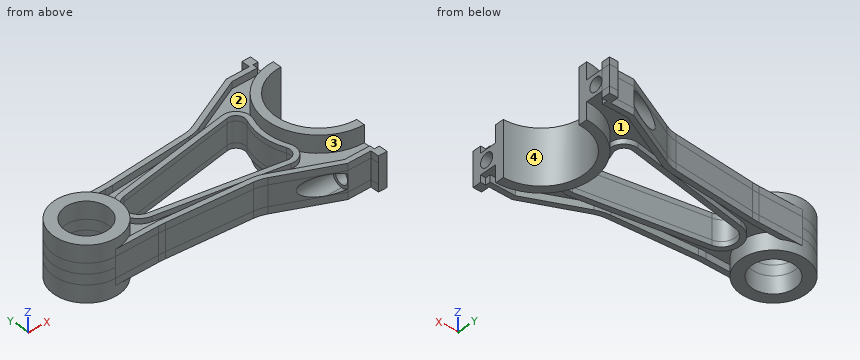
from build123d import *

# Parameters (mm, degrees)
SKETCH1_R           = 19
SKETCH1_R_2         = 12.5
BOSS_EXTRUDE1_DEPTH = 6
SKETCH1_4_R         = 19
SKETCH1_4_R_2       = 12.5
BOSS_EXTRUDE2_DEPTH = 16
BOSS_EXTRUDE3_DEPTH = 10
SKETCH3_R           = 4
CUT_EXTRUDE2_DEPTH  = 18.5
SKETCH4_R           = 5.795
CUT_EXTRUDE4_DEPTH  = 144.94417008
BOSS_EXTRUDE4_DEPTH = 9


with BuildPart() as part:
    # Sketch1 → Boss-Extrude1 (new, symmetric)
    # profile 1 of 3: a face of its own
    with BuildSketch(Plane.XY):
        with Locations((-135.29, 0)):
            Circle(SKETCH1_R)
        with Locations((-135.29, 0)):
            Circle(SKETCH1_R_2, mode=Mode.SUBTRACT)
    # profile 2 of 3: a face of its own
    with BuildSketch(Plane.XY):
        with BuildLine():
            Line((-110.00450535, 19), (-135.29, 19))
            ThreePointArc((-135.29, 19), (-121.854971157, 13.435028843), (-116.29, 0))
            ThreePointArc((-116.29, 0), (-121.854971157, -13.435028843), (-135.29, -19))
            Line((-135.29, -19), (-110.00450535, -19))
            ThreePointArc((-110.00450535, -19), (-108.041514562, -19.038548188), (-106.081550564, -19.154133313))
            Line((-106.081550564, -19.154133313), (-58.361460534, -22.909785849))
            ThreePointArc((-58.361460534, -22.909785849), (-54.838603484, -23.507213745), (-51.478277214, -24.721976782))
            Line((-51.478277214, -24.721976782), (-18.5, -40.1))
            Line((-18.5, -40.1), (-5, -40.1))
            Line((-5, -40.1), (-5, -45))
            Line((-5, -45), (0, -45))
            Line((0, -45), (0, -30))
            ThreePointArc((0, -30), (-30, 0), (0, 30))
            Line((0, 30), (0, 45))
            Line((0, 45), (-5, 45))
            Line((-5, 45), (-5, 40.1))
            Line((-5, 40.1), (-18.5, 40.1))
            Line((-18.5, 40.1), (-51.478277214, 24.721976782))
            ThreePointArc((-51.478277214, 24.721976782), (-54.838603484, 23.507213745), (-58.361460534, 22.909785849))
            Line((-58.361460534, 22.909785849), (-106.081550564, 19.154133313))
            ThreePointArc((-106.081550564, 19.154133313), (-108.041514562, 19.038548188), (-110.00450535, 19))
        make_face()
        with BuildLine():
            ThreePointArc((-106.341033016, -7.886801028), (-113, 0), (-106.341033016, 7.886801028))
            Line((-106.341033016, 7.886801028), (-35.770781366, 19.886220952))
            ThreePointArc((-35.770781366, 19.886220952), (-31.0052687, 18.051447358), (-30.336236293, 12.988947901))
            ThreePointArc((-30.336236293, 12.988947901), (-33, 0), (-30.336236293, -12.988947901))
            ThreePointArc((-30.336236293, -12.988947901), (-31.0052687, -18.051447358), (-35.770781366, -19.886220952))
            Line((-35.770781366, -19.886220952), (-106.341033016, -7.886801028))
        make_face(mode=Mode.SUBTRACT)
    # profile 3 of 3: a face of its own
    with BuildSketch(Plane.XY):
        with BuildLine():
            Line((0, 25), (0, 30))
            ThreePointArc((0, 30), (-30, 0), (0, -30))
            Line((0, -30), (0, -25))
            ThreePointArc((0, -25), (-25, 0), (0, 25))
        make_face()
    extrude(amount=BOSS_EXTRUDE1_DEPTH, both=True)

    # Sketch1_4 → Boss-Extrude2 (add, symmetric)
    # profile 1 of 2: a face of its own
    with BuildSketch(Plane.XY):
        with Locations((-135.29, 0)):
            Circle(SKETCH1_4_R)
        with Locations((-135.29, 0)):
            Circle(SKETCH1_4_R_2, mode=Mode.SUBTRACT)
    # profile 2 of 2: a face of its own
    with BuildSketch(Plane.XY):
        with BuildLine():
            Line((0, 25), (0, 30))
            ThreePointArc((0, 30), (-30, 0), (0, -30))
            Line((0, -30), (0, -25))
            ThreePointArc((0, -25), (-25, 0), (0, 25))
        make_face()
    extrude(amount=BOSS_EXTRUDE2_DEPTH, both=True)

    # Sketch2 → Boss-Extrude3 (add, symmetric)
    with BuildSketch(Plane.XY):
        with BuildLine():
            Line((-5, 45), (-5, 40.1))
            Line((-5, 40.1), (-18.5, 40.1))
            Line((-18.5, 40.1), (-51.478277214, 24.721976782))
            ThreePointArc((-51.478277214, 24.721976782), (-54.838603484, 23.507213745), (-58.361460534, 22.909785849))
            Line((-58.361460534, 22.909785849), (-106.081550564, 19.154133313))
            ThreePointArc((-106.081550564, 19.154133313), (-108.041514562, 19.038548188), (-110.00450535, 19))
            Line((-110.00450535, 19), (-135.29, 19))
            ThreePointArc((-135.29, 19), (-129.951460874, 18.234582529), (-125.043049234, 16))
            Line((-125.043049234, 16), (-110.00450535, 16))
            ThreePointArc((-110.00450535, 16), (-107.923735115, 16.040861079), (-105.846173277, 16.163381312))
            Line((-105.846173277, 16.163381312), (-58.126083247, 19.919033847))
            ThreePointArc((-58.126083247, 19.919033847), (-54.07479764, 20.606075928), (-50.210422429, 22.003053421))
            Line((-50.210422429, 22.003053421), (-17.834916012, 37.1))
            Line((-17.834916012, 37.1), (-3, 37.1))
            Line((-3, 37.1), (-3, 40))
            Line((-3, 40), (0, 40))
            Line((0, 40), (0, 45))
            Line((0, 45), (-5, 45))
        make_face()
        with BuildLine():
            Line((0, -40), (-3, -40))
            Line((-3, -40), (-3, -37.1))
            Line((-3, -37.1), (-17.834916012, -37.1))
            Line((-17.834916012, -37.1), (-50.210422429, -22.003053421))
            ThreePointArc((-50.210422429, -22.003053421), (-54.07479764, -20.606075928), (-58.126083247, -19.919033847))
            Line((-58.126083247, -19.919033847), (-105.846173277, -16.163381312))
            ThreePointArc((-105.846173277, -16.163381312), (-107.923735115, -16.040861079), (-110.00450535, -16))
            Line((-110.00450535, -16), (-125.043049234, -16))
            ThreePointArc((-125.043049234, -16), (-129.951460874, -18.234582529), (-135.29, -19))
            Line((-135.29, -19), (-110.00450535, -19))
            ThreePointArc((-110.00450535, -19), (-108.041514562, -19.038548188), (-106.081550564, -19.154133313))
            Line((-106.081550564, -19.154133313), (-58.361460534, -22.909785849))
            ThreePointArc((-58.361460534, -22.909785849), (-54.838603484, -23.507213745), (-51.478277214, -24.721976782))
            Line((-51.478277214, -24.721976782), (-18.5, -40.1))
            Line((-18.5, -40.1), (-5, -40.1))
            Line((-5, -40.1), (-5, -45))
            Line((-5, -45), (0, -45))
            Line((0, -45), (0, -40))
        make_face()
    extrude(amount=BOSS_EXTRUDE3_DEPTH, both=True)

    # Sketch3 → Cut-Extrude2 (cut)
    with BuildSketch(Plane(origin=(0, 0, 0), x_dir=(0, 0, -1), z_dir=(1, 0, 0))):
        with Locations(Location((0, -36, 0), (0, 0, 90))):
            Circle(SKETCH3_R)
    cut_extrude2 = extrude(amount=-CUT_EXTRUDE2_DEPTH, mode=Mode.SUBTRACT)

    # Sketch4 → Cut-Extrude4 (cut, through all)
    with BuildSketch(Plane(origin=(-18.5, 0, 0), x_dir=(0, 0, -1), z_dir=(1, 0, 0))):
        with Locations((0, -36)):
            Circle(SKETCH4_R)
    cut_extrude4 = extrude(amount=-CUT_EXTRUDE4_DEPTH, mode=Mode.SUBTRACT)

    # Mirror1: Cut-Extrude2, Cut-Extrude4 across plane
    add(cut_extrude2.mirror(Plane.ZX), mode=Mode.SUBTRACT)
    add(cut_extrude4.mirror(Plane.ZX), mode=Mode.SUBTRACT)

    # Sketch5 → Boss-Extrude4 (add, symmetric)
    with BuildSketch(Plane.XY):
        with BuildLine():
            Line((-106.843920397, 10.844351413), (-36.273668747, 22.843771338))
            ThreePointArc((-36.273668747, 22.843771338), (-28.648848481, 19.908133587), (-27.57839663, 11.808134455))
            ThreePointArc((-27.57839663, 11.808134455), (-30, 0), (-27.57839663, -11.808134455))
            ThreePointArc((-27.57839663, -11.808134455), (-28.648848481, -19.908133587), (-36.273668747, -22.843771338))
            Line((-36.273668747, -22.843771338), (-106.843920397, -10.844351413))
            ThreePointArc((-106.843920397, -10.844351413), (-116, 0), (-106.843920397, 10.844351413))
        make_face()
        with BuildLine():
            Line((-106.341033016, -7.886801028), (-35.770781366, -19.886220952))
            ThreePointArc((-35.770781366, -19.886220952), (-31.0052687, -18.051447358), (-30.336236293, -12.988947901))
            ThreePointArc((-30.336236293, -12.988947901), (-33, 0), (-30.336236293, 12.988947901))
            ThreePointArc((-30.336236293, 12.988947901), (-31.0052687, 18.051447358), (-35.770781366, 19.886220952))
            Line((-35.770781366, 19.886220952), (-106.341033016, 7.886801028))
            ThreePointArc((-106.341033016, 7.886801028), (-113, 0), (-106.341033016, -7.886801028))
        make_face(mode=Mode.SUBTRACT)
    extrude(amount=BOSS_EXTRUDE4_DEPTH, both=True)


solid = part.part
Read the model definition and answer for the solid it produces. Units are mm, in the model's axes. Face numbers are marked on the shaded views. A direction names the side the tool comes from. Coordinates: 2 decimals unless noted, no trailing zeros. Write each loop counter-clockwise with the first axis right and the second up, starting at its lowest first coordinate (ties: lowest second). Pieces come first, ordered by that corner, then holes. Notation, with made-up numbers: (80, 8) -> (135, 8) arc R22 ccw to (135, 39) -> close; hole circle Ø4 at (-0.75, -17). An arc over 180 degrees is marked (long way). Return JSON: item names as keys, results as strings.
(1) The part is cut by section A-A on y = 0. Give the vertices of the cut face in (x, z).
Answers below:
{"outline": "(-154.29, -16) -> (-147.79, -16) -> (-147.79, 16) -> (-154.29, 16) -> close; (-122.79, -16) -> (-116.29, -16) -> (-116.29, -6) -> (-116, -6) -> (-116, -9) -> (-113, -9) -> (-113, 9) -> (-116, 9) -> (-116, 6) -> (-116.29, 6) -> (-116.29, 16) -> (-122.79, 16) -> close; (-33, -9) -> (-30, -9) -> (-30, -16) -> (-25, -16) -> (-25, 16) -> (-30, 16) -> (-30, 9) -> (-33, 9) -> close"}
(2) The part is cut by section C-C on x = -111.5. Give the vertices of the cut face in (y, z).
Answers below:
{"outline": "(-19, -10) -> (-16, -10) -> (-16, -6) -> (-8.87, -6) -> (-8.87, -9) -> (-4.66, -9) -> (-4.66, 9) -> (-8.87, 9) -> (-8.87, 6) -> (-16, 6) -> (-16, 10) -> (-19, 10) -> close; (4.66, -9) -> (8.87, -9) -> (8.87, -6) -> (16, -6) -> (16, -10) -> (19, -10) -> (19, 10) -> (16, 10) -> (16, 6) -> (8.87, 6) -> (8.87, 9) -> (4.66, 9) -> close"}
(3) For a pull along X with two mould halves and no side action, classify the marked faces 3 and 4 as pulls with the +X half, pulls with the -X half, needs draft (parallel to the pull), parting line crosses it, or undercut.
Answers below:
{"face 3": "undercut", "face 4": "pulls with the +X half"}
(4) Which of the six approach directions +Z, -Z, +X, -X, +Y, -Y give full straight-line access (tool end or side, diameter ignored) to the marked faces 1 and 2?
Answers below:
{"face 1": "-Z", "face 2": "+Z"}
(5) Consider line 1 along Z through (x, y) = (-11, 36); line 2 along Y through (x, z) = (-135.29, -10); line 3 along X through (y, z) = (11, -10). Determine where each line is inside the solid, lowest interval first. Write a range as from..to.
Answers below:
{"line 1": "-6..-4, 4..6", "line 2": "-19..-12.5, 12.5..19", "line 3": "-150.78..-141.23, -129.35..-119.8, -27.91..-22.45"}
(6) Each of these flat-tipped pins is pushed along its axis until it touches: P1, Ø5, axis at y = 9, z = -1, coming from the -X side; P2, Ø2, axis at x = -13.5, z = -8, coming from the -Y side; P3, Ø4.5, axis at y = -42.5, z = 8, coming from the -X side; P4, Ø22.5, axis at x = -135.29, y = 0, coming from the +Z side. Where does it stop, or does it pass through?
Answers below:
{"P1": "x = -153.14", "P2": "y = -40.1", "P3": "x = -5", "P4": "through"}
(7) The part is cut by section B-B on z = 13. Give the vertices of the cut face in (x, y).
Answers below:
{"outline": "circle Ø38 at (-135.29, 0); (0, -30) -> (0, -25) arc R25 cw to (0, 25) -> (0, 30) arc R30 ccw to start; hole circle Ø25 at (-135.29, 0)"}
